Design review of the part built by this model. Coordinates are the model's own, in mm. A direction names the side the tool comes from. Give positions to 0.01 mm unless a question says otherwise; leave off trailing zeros. Write each loop counter-clockwise with the first axis right and the second up, starting at its lowest first coordinate (ties: lowest second). Pieces come first, ordered by that corner, then holes. Notation, with made-up numbers: (25, 82.25) -> (39, 82.25) arc R16 cw to (39, 94.25) -> close; hole circle Ø9 at (44, 23.25). An arc over 180 degrees is marked (long way). Write each question's results on one line, items separated by ' | '. Start each with the question number.
(1) Clearance check with flat-ended pins moving along their axes: pin 1 (0.6 mm diameter, centred on y = 1, z = 4, fed in from -X); pin 2 (4 mm diameter, centred on x = 7, z = -11, fed in from +Y); pin 3 (1 mm diameter, centred on x = 11, y = 0.5, fed in from +Z). State where each tip first meets the part, or that it passes through.
(2) Take a section at A-A (z = 11.5). State the section outline as (x, y) points.
(3) Take a section at D-D (x = 14). State the section outline as (y, z) points, plus the area to 3 significant figures.
(4) Mouldability with a two-part tool opening along Z and no side actions: class faces 4 (the face through (-5.541, 0.986, -1.874)), 5 (the face through (10.5, 1, -10)), 6 (the face through (-16.347, 1.014, 15.104)) as released by +Z, released by -Z, zero draft, split by the parting line, or undercut.
(5) To check wall thickness, follow probe 1 along X at (y, z) = (0.8, -10.5); probe 2 along X at (y, z) = (0.85, 13.5); probe 3 along X at (y, z) = (0.15, -0.5). State the ranges of each line that lie inside material, in increasing order.
(6) Take a section at B-B (x = 21). State the section outline as (y, z) points, plus the area to 3 significant figures.
(7) For faces 1 (the face through (-10.5, 1, -9)), 2 (the face through (16.31, 1.01, 15.07)), 3 (the face through (5.569, 0.986, -1.884)), list the 3-axis set-ups (+Z, -Z, +X, -X, +Y, -Y) from which the entire face can be reached by the end or side of a thin tool; tool diameter is ignored.
(8) Take a section at C-C (y = 0.6). Count the separate pieces of the cut face and the enclosed holes in it, plus the area to 3 significant figures.
from build123d import *

# Parameters (mm, degrees)
SKETCH1_R             = 1.5
BOSS_EXTRUDE1_DEPTH   = 2
SKETCH2_R             = 3.5
BOSS_EXTRUDE2_DEPTH   = 2
SKETCH3_R             = 1.5
CUT_EXTRUDE1_DEPTH    = 2
SKETCH4_R             = 1.5
CUT_EXTRUDE2_DEPTH    = 2
BOSS_EXTRUDE3_START   = -2
BOSS_EXTRUDE3_DEPTH   = 2
SKETCH8_R             = 4
BOSS_EXTRUDE5_DEPTH   = 2
SKETCH9_R             = 1.5
CUT_EXTRUDE4_DEPTH    = 2
CUT_EXTRUDE5_DEPTH    = 2
BOSS_EXTRUDE12_DEPTH  = 2
CUT_EXTRUDE11_DEPTH   = 2
CUT_EXTRUDE15_DEPTH   = 19
FILLET1_R             = 5
FILLET2_R             = 4
FILLET1_OF_MIRROR13_R = 5
FILLET2_OF_MIRROR13_R = 4


with BuildPart() as part:
    # Sketch1 → Boss-Extrude1 (new body)
    # profile 1 of 5: a face of its own
    with BuildSketch(Plane(origin=(0, 0, 0), x_dir=(1, 0, 0), z_dir=(0, 1, 0))):
        with BuildLine():
            Line((20.5, 14), (10.5, 14))
            Line((10.5, 14), (10.5, 5))
            Line((10.5, 5), (-10.5, 5))
            Line((-10.5, 5), (-10.5, 14))
            Line((-10.5, 14), (-20.5, 14))
            Line((-20.5, 14), (-20.5, -14))
            ThreePointArc((-20.5, -14), (0, -5.789884137), (20.5, -14))
            Line((20.5, -14), (20.5, 7))
            ThreePointArc((20.5, 7), (17, 10.5), (20.5, 14))
        make_face()
        with Locations(Location((13.5, 10.5, 0), (0, 0, 270))):
            Circle(SKETCH1_R, mode=Mode.SUBTRACT)
    # profile 2 of 5: a face of its own
    with BuildSketch(Plane(origin=(0, 0, 0), x_dir=(1, 0, 0), z_dir=(0, 1, 0))):
        with BuildLine():
            ThreePointArc((24, 10.5), (22.974873734, 12.974873734), (20.5, 14))
            Line((20.5, 14), (20.5, 12))
            ThreePointArc((20.5, 12), (21.560660172, 11.560660172), (22, 10.5))
            ThreePointArc((22, 10.5), (21.560660172, 9.439339828), (20.5, 9))
            Line((20.5, 9), (20.5, 7))
            ThreePointArc((20.5, 7), (22.974873734, 8.025126266), (24, 10.5))
        make_face()
    # profile 3 of 5: a face of its own
    with BuildSketch(Plane(origin=(0, 0, 0), x_dir=(1, 0, 0), z_dir=(0, 1, 0))):
        with BuildLine():
            Line((20.5, 12), (20.5, 14))
            ThreePointArc((20.5, 14), (17, 10.5), (20.5, 7))
            Line((20.5, 7), (20.5, 9))
            ThreePointArc((20.5, 9), (19, 10.5), (20.5, 12))
        make_face()
    # profile 4 of 5: a face of its own
    with BuildSketch(Plane(origin=(0, 0, 0), x_dir=(1, 0, 0), z_dir=(0, 1, 0))):
        with BuildLine():
            ThreePointArc((24, 10.5), (22.974873734, 12.974873734), (20.5, 14))
            Line((20.5, 14), (20.5, 12))
            ThreePointArc((20.5, 12), (21.560660172, 11.560660172), (22, 10.5))
            ThreePointArc((22, 10.5), (21.560660172, 9.439339828), (20.5, 9))
            Line((20.5, 9), (20.5, 7))
            ThreePointArc((20.5, 7), (22.974873734, 8.025126266), (24, 10.5))
        make_face()
    # profile 5 of 5: a face of its own
    with BuildSketch(Plane(origin=(0, 0, 0), x_dir=(1, 0, 0), z_dir=(0, 1, 0))):
        with BuildLine():
            Line((20.5, 12), (20.5, 14))
            ThreePointArc((20.5, 14), (17, 10.5), (20.5, 7))
            Line((20.5, 7), (20.5, 9))
            ThreePointArc((20.5, 9), (19, 10.5), (20.5, 12))
        make_face()
    extrude(amount=BOSS_EXTRUDE1_DEPTH)

    # Sketch2 → Boss-Extrude2 (add)
    with BuildSketch(Plane(origin=(0, 2, 0), x_dir=(1, 0, 0), z_dir=(0, 1, 0))):
        with Locations((-20.5, 10.5)):
            Circle(SKETCH2_R)
    extrude(amount=-BOSS_EXTRUDE2_DEPTH)

    # Sketch3 → Cut-Extrude1 (cut)
    with BuildSketch(Plane(origin=(0, 2, 0), x_dir=(1, 0, 0), z_dir=(0, 1, 0))):
        with Locations(Location((-20.5, 10.5, 0), (0, 0, 270))):
            Circle(SKETCH3_R)
    extrude(amount=-CUT_EXTRUDE1_DEPTH, mode=Mode.SUBTRACT)

    # Sketch4 → Cut-Extrude2 (cut)
    with BuildSketch(Plane(origin=(0, 2, 0), x_dir=(1, 0, 0), z_dir=(0, 1, 0))):
        with Locations(Location((-13.5, 10.5, 0), (0, 0, 270))):
            Circle(SKETCH4_R)
    extrude(amount=-CUT_EXTRUDE2_DEPTH, mode=Mode.SUBTRACT)

    # Sketch5 → Boss-Extrude3 (add)
    with BuildSketch(Plane(origin=(0, 2, 0), x_dir=(1, 0, 0), z_dir=(0, 1, 0)).offset(BOSS_EXTRUDE3_START)):
        with BuildLine():
            Line((-20.5, -14), (20.5, -14))
            ThreePointArc((20.5, -14), (0, -5.789884137), (-20.5, -14))
        make_face()
    extrude(amount=BOSS_EXTRUDE3_DEPTH)

    # Sketch8 → Boss-Extrude5 (add)
    with BuildSketch(Plane(origin=(0, 2, 0), x_dir=(1, 0, 0), z_dir=(0, 1, 0))):
        with Locations((20.5, -13.5)):
            Circle(SKETCH8_R)
    boss_extrude5 = extrude(amount=-BOSS_EXTRUDE5_DEPTH)

    # Sketch9 → Cut-Extrude4 (cut)
    with BuildSketch(Plane(origin=(0, 2, 0), x_dir=(1, 0, 0), z_dir=(0, 1, 0))):
        with Locations(Location((20.5, -13.5, 0), (0, 0, 270))):
            Circle(SKETCH9_R)
    cut_extrude4 = extrude(amount=-CUT_EXTRUDE4_DEPTH, mode=Mode.SUBTRACT)

    # Sketch10 → Cut-Extrude5 (cut)
    with BuildSketch(Plane(origin=(0, 2, 0), x_dir=(1, 0, 0), z_dir=(0, 1, 0))):
        with BuildLine():
            Line((20.5, 7), (20.5, -9.5))
            ThreePointArc((20.5, -9.5), (17.08273811, -1.25), (20.5, 7))
        make_face()
    cut_extrude5 = extrude(amount=-CUT_EXTRUDE5_DEPTH, mode=Mode.SUBTRACT)

    # Mirror12: Boss-Extrude5, Cut-Extrude4, Cut-Extrude5 across plane
    add(boss_extrude5.mirror(Plane(origin=(0, 0, 0), x_dir=(0, 0, 1), z_dir=(1, 0, 0))))
    add(cut_extrude4.mirror(Plane(origin=(0, 0, 0), x_dir=(0, 0, 1), z_dir=(1, 0, 0))), mode=Mode.SUBTRACT)
    add(cut_extrude5.mirror(Plane(origin=(0, 0, 0), x_dir=(0, 0, 1), z_dir=(1, 0, 0))), mode=Mode.SUBTRACT)

    # Sketch12 → Boss-Extrude12 (add)
    with BuildSketch(Plane(origin=(0, 2, 0), x_dir=(1, 0, 0), z_dir=(0, 1, 0))):
        with BuildLine():
            Line((-14.965299889, -14), (-16.531373033, -14))
            ThreePointArc((-16.531373033, -14), (-16.889121467, -15.220917262), (-17.61216057, -16.267739768))
            ThreePointArc((-17.61216057, -16.267739768), (-16.328147274, -15.087863095), (-14.965299889, -14))
        make_face()
        with BuildLine():
            Line((16.531373033, -14), (14.965299889, -14))
            ThreePointArc((14.965299889, -14), (16.328147274, -15.087863095), (17.61216057, -16.267739768))
            ThreePointArc((17.61216057, -16.267739768), (16.889121467, -15.220917262), (16.531373033, -14))
        make_face()
    extrude(amount=-BOSS_EXTRUDE12_DEPTH)

    # Sketch20 → Cut-Extrude11 (cut)
    with BuildSketch(Plane(origin=(0, 2, 0), x_dir=(1, 0, 0), z_dir=(0, 1, 0))):
        with BuildLine():
            Line((14.965299889, -14), (-14.965299889, -14))
            ThreePointArc((-14.965299889, -14), (0, -9.149002287), (14.965299889, -14))
        make_face()
    extrude(amount=-CUT_EXTRUDE11_DEPTH, mode=Mode.SUBTRACT)

    # Sketch21 → Cut-Extrude15 (cut)
    with BuildSketch(Plane(origin=(0, 2, 0), x_dir=(1, 0, 0), z_dir=(0, 1, 0))):
        Polygon((11.539683191, 2.764795759), (2.206859121, 1.551865555), (2.206859121, -5.254020589), (11.539683191, -6.904953367), (11.539683191, -2.592312642), align=None)
    cut_extrude15 = extrude(amount=-CUT_EXTRUDE15_DEPTH, mode=Mode.SUBTRACT)

    # Fillet1
    fillet1_edges = [part.edges().sort_by_distance(p)[0] for p in [
        (2.206859121, 1, -1.551865555),
    ]]
    fillet(fillet1_edges, radius=FILLET1_R)

    # Fillet2
    fillet2_edges = [part.edges().sort_by_distance(p)[0] for p in [
        (2.206859121, 1, 5.254020589),
    ]]
    fillet(fillet2_edges, radius=FILLET2_R)

    # Mirror13: Cut-Extrude15 across plane
    add(cut_extrude15.mirror(Plane(origin=(0, 0, 0), x_dir=(0, 0, 1), z_dir=(1, 0, 0))), mode=Mode.SUBTRACT)

    # Fillet1 of Mirror13
    fillet1_of_mirror13_edges = [part.edges().sort_by_distance(p)[0] for p in [
        (-2.206859121, 1, -1.551865555),
    ]]
    fillet(fillet1_of_mirror13_edges, radius=FILLET1_OF_MIRROR13_R)

    # Fillet2 of Mirror13
    fillet2_of_mirror13_edges = [part.edges().sort_by_distance(p)[0] for p in [
        (-2.206859121, 1, 5.254020589),
    ]]
    fillet(fillet2_of_mirror13_edges, radius=FILLET2_OF_MIRROR13_R)


solid = part.part
Report:
1) pin 1: x = -17.49 | pin 2: through | pin 3: z = 11.89
2) outline: (-23.96, 0) -> (-10.7, 0) -> (-10.7, 2) -> (-23.96, 2) -> close; (10.7, 0) -> (23.96, 0) -> (23.96, 2) -> (10.7, 2) -> close
3) outline: (0, -14) -> (2, -14) -> (2, -11.91) -> (0, -11.91) -> close; (0, -9.09) -> (2, -9.09) -> (2, 13.33) -> (0, 13.33) -> close | area: 49.0 mm2
4) face 4: undercut | face 5: zero draft | face 6: released by +Z
5) probe 1: -24 to -22, -19 to -15, -12 to -10.5, 10.5 to 12, 15 to 19, 22 to 24 | probe 2: -24.5 to -22, -19 to -14.25, 14.25 to 19, 22 to 24.5 | probe 3: -17.21 to -11.54, -3.55 to 3.55, 11.54 to 17.21
6) outline: (0, -13.96) -> (2, -13.96) -> (2, -11.91) -> (0, -11.91) -> close; (0, -9.09) -> (2, -9.09) -> (2, -7.04) -> (0, -7.04) -> close; (0, 9.53) -> (2, 9.53) -> (2, 12.09) -> (0, 12.09) -> close; (0, 14.91) -> (2, 14.91) -> (2, 17.47) -> (0, 17.47) -> close | area: 18.4 mm2
7) face 1: -Z, +Y, -Y | face 2: +Z, +Y, -Y | face 3: +Y, -Y
8) separate pieces: 1 | enclosed holes: 8 | area: 716 mm2
